from build123d import *

# Parameters (mm, degrees)
F1_R      = 30
F2_DEPTH  = 16
F3_DEPTH  = 13
F4_R      = 6.5
F5_DEPTH  = 16.001
F6_R      = 2.5
F7_DEPTH  = 16.001
F8_R      = 5
F9_R      = 27.5
F9_R_2    = 10
F9_R_3    = 5
F10_DEPTH = 11
F11_DEPTH = 3


with BuildPart() as f2:
    # F1 (on Top) → F2 (new body)
    with BuildSketch(Plane.XY):
        Circle(F1_R)
    extrude(amount=F2_DEPTH)

    # F0 (on Top) → F3 (cut)
    with BuildSketch(Plane.XY):
        Polygon((0.5, 7.4833147735), (0.5, 6.4807406984), (-0.5, 6.4807406984), (-0.5, 7.4833147735), (-2.0895980578, 7.2030257501), (-1.746697532, 6.2609142888), (-2.6863901539, 5.9188941485), (-3.0292906797, 6.8610056098), (-4.4271597759, 6.0539455166), (-3.782717585, 5.2859292156), (-4.54876203, 4.6431416082), (-5.193204221, 5.4111579093), (-6.2307406865, 4.1746701064), (-5.3624860697, 3.6733830663), (-5.8624860722, 2.807357664), (-6.730740689, 3.308644704), (-7.2828023136, 1.7918678691), (-6.2954595919, 1.6177727054), (-6.4691077722, 0.6329649529), (-7.4564504939, 0.8070601166), (-7.456450498, -0.8070600785), (-6.4691077754, -0.6329649198), (-6.2954596002, -1.6177726732), (-7.2828023228, -1.7918678319), (-6.7307407059, -3.3086446696), (-5.8624860865, -2.807357634), (-5.3624860885, -3.6733830389), (-6.2307407079, -4.1746700745), (-5.1932042487, -5.4111578827), (-4.5487620538, -4.643141585), (-3.782717612, -5.2859291963), (-4.4271598069, -6.053945494), (-3.0292907148, -6.8610055943), (-2.6863901841, -5.9188941348), (-1.746697564, -6.2609142799), (-2.0895980946, -7.2030257394), (-0.5000000128, -7.4833147727), (-0.500000011, -6.4807406976), (0.499999989, -6.4807406993), (0.4999999872, -7.4833147744), (2.0895980701, -7.2030257465), (1.7466975426, -6.2609142858), (2.686390164, -5.9188941439), (3.0292906914, -6.8610056046), (4.4271597862, -6.0539455091), (3.782717594, -5.2859292092), (4.5487620379, -4.6431416005), (5.1932042302, -5.4111579004), (6.2307406937, -4.1746700957), (5.362486076, -3.6733830572), (5.862486077, -2.807357654), (6.7307406946, -3.3086446925), (7.2828023167, -1.7918678567), (6.2954595947, -1.6177726947), (6.4691077733, -0.6329649418), (7.4564504953, -0.8070601039), (7.4564504967, 0.8070600912), (6.4691077744, 0.6329649308), (6.2954595974, 1.6177726839), (7.2828023197, 1.7918678443), (6.7307407003, 3.3086446811), (5.8624860818, 2.807357644), (5.3624860822, 3.673383048), (6.2307407008, 4.1746700851), (5.1932042394, 5.4111578916), (4.5487620458, 4.6431415927), (3.782717603, 5.2859292027), (4.4271597966, 6.0539455016), (3.0292907031, 6.8610055995), (2.686390174, 5.9188941393), (1.7466975533, 6.2609142829), (2.0895980824, 7.203025743), align=None)
    extrude(amount=F3_DEPTH, mode=Mode.SUBTRACT)

    # F4 (on Top) → F5 (cut, through all)
    with BuildSketch(Plane.XY):
        Circle(F4_R)
    extrude(amount=F5_DEPTH, mode=Mode.SUBTRACT)

    # F6 (on Top) → F7 (cut, through all)
    with BuildSketch(Plane.XY):
        with Locations((20, 0)):
            Circle(F6_R)
    extrude(amount=F7_DEPTH, mode=Mode.SUBTRACT)

    # F8
    f8_edges = [f2.edges().sort_by_distance(p)[0] for p in [
        (-30, 0, 16),
    ]]
    fillet(f8_edges, radius=F8_R)

    # F9 (on Top) → F10 (cut)
    with BuildSketch(Plane.XY):
        Circle(F9_R)
        Circle(F9_R_2, mode=Mode.SUBTRACT)
        with Locations((20, 0)):
            Circle(F9_R_3, mode=Mode.SUBTRACT)
    extrude(amount=F10_DEPTH, mode=Mode.SUBTRACT)

    # F11 (cut): a face of the model
    f11_faces = [f2.faces().sort_by_distance(p)[0] for p in [
        (15.1414213562, 0, 0),
    ]]
    extrude(f11_faces, amount=-F11_DEPTH, mode=Mode.SUBTRACT)


solid = f2.part
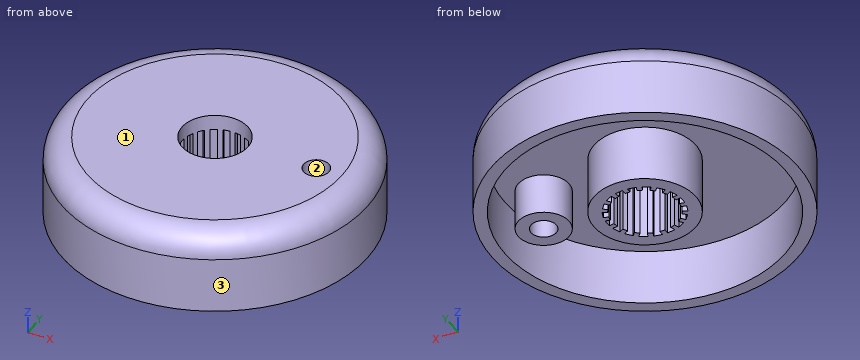
Geometry: final body of the model. Coordinates: model frame, mm. Face numbers are marked on the shaded views. Coordinates: 2 decimals unless noted, no trailing zeros.
(1) Draft query along X for the marked faces 1, 2 and 3. Return one class per face: pulls with the +X half, pulls with the -X half, needs draft (parallel to the pull), parting line crosses it, or undercut.
(2) Section query A-A (z = 5.5). State how many separate pieces and enclosed holes the cut face has, plus the area to 3 significant figures.
(3) Material intervals for probe 1 along Y at (x, z) = (0, 3.5); probe 2 along X at (y, z) = (-2.5, 1.75); probe 3 along Y at (x, z) = (20, 8.5), sorted ascending.
(4) First-contact query: pin 1 (0.7 mm diameter, centred on x = -6.5, y = -2.5, fed in from -Z); pin 2 (1.5 mm diameter, centred on x = 2.5, z = 10, fed in from +Y); pin 3 (2 mm diameter, centred on x = -17.5, z = 1.5, fed in from +Y); pin 4 (8 mm diameter, centred on x = 0, y = 0, fed in from +Z). Flat tips, straight axial feed; report the tip coordinate or a pass-through.
Solution:
1. face 1: needs draft
1. face 2: undercut
1. face 3: parting line crosses it
2. separate pieces: 3
2. enclosed holes: 3
2. area: 667 mm2
3. probe 1: y = -30 to -27.5, -10 to -6.5, 6.5 to 10, 27.5 to 30
3. probe 2: x = -29.9 to -27.39, -9.68 to -7.03, 7.03 to 9.68, 27.39 to 29.9
3. probe 3: y = -22.36 to -18.87, -5 to -2.5, 2.5 to 5, 18.87 to 22.36
4. pin 1: stops at z = 13
4. pin 2: stops at y = 29.95
4. pin 3: stops at y = 25.05
4. pin 4: passes through
